Can you work these out from the model? Positions are in its coordinate system, mm. Face numbers are marked on the shaded views. A direction names the side the tool comes from. Coordinates: 2 decimals unless noted, no trailing zeros. Order: outer loops, then holes, each group sorted by start corner. A loop starts at its lowest first (then second) coordinate and runs counter-clockwise, first axis right, second up.
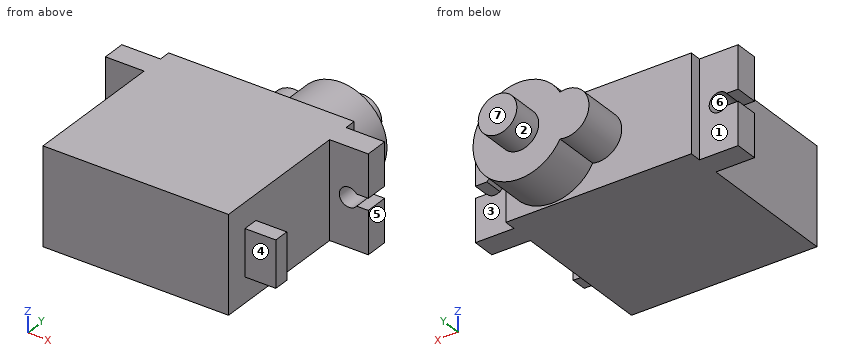
Autodesk Inventor part; units mm, degrees
ref_plane "YZ Plane" through (0, 0, 0) normal (1, 0, 0) x (0, 1, 0)
ref_plane "XZ Plane" through (0, 0, 0) normal (0, 1, 0) x (-1, 0, 0)
ref_plane "XY Plane" through (0, 0, 0) normal (0, 0, 1) x (1, 0, 0)
sketch "草圖1" plane through (0, 0, 0) normal (0, 0, 1) x (1, 0, 0)
  line L0 (-18, -14.5) -> (6, -14.5)
  line L1 (6, -14.5) -> (6, -33)
  line L2 (6, -33) -> (-18, -33)
  line L3 (-18, -33) -> (-18, -14.5)
  line L4 (-23, -11.5) -> (11, -11.5)
  line L5 (11, -11.5) -> (11, -14.5)
  line L6 (11, -14.5) -> (-23, -14.5)
  line L7 (-23, -14.5) -> (-23, -11.5)
  line L8 (6, -11.5) -> (-18, -11.5)
  line L9 (-18, -11.5) -> (-18, -10)
  line L10 (-18, -10) -> (6, -10)
  line L11 (6, -10) -> (6, -11.5)
  line L12 (6, -10) -> (-9, -10)
  line L13 (-9, -10) -> (-9, -4)
  line L14 (-9, -4) -> (6, -4)
  line L15 (6, -4) -> (6, -10)
  line L16 (2.5, -4) -> (-2.5, -4)
  line L17 (-2.5, -4) -> (-2.5, 0)
  line L18 (-2.5, 0) -> (2.5, 0)
  line L19 (2.5, 0) -> (2.5, -4)
  point P0 (0, 0)
  point P1 (-6, -14.5)
  point P2 (-6, -11.5)
  point P3 (0, -4)
  point P4 (-18, -11.5)
  point P5 (6, -14.5)
  point P6 (0, 0)
  dimension "d0" = 24
  dimension "d1" = 18.5
  dimension "d2" = 34
  dimension "d3" = 3
  dimension "d4" = 1.5
  dimension "d5" = 6
  dimension "d6" = 9
  dimension "d7" = 5
  dimension "d8" = 4
  dimension "d9" = 6
extrude "擠出1" add sketch "草圖1" along normal mid plane 12.5 contours L6 L7 L4 L5 L0 | L0 L1 L2 L3 | L9 L10 L11 L4
sketch "草圖2" plane through (-18, -10, 6.25) normal (0, 1, 0) x (1, 0, 0)
  circle A0 centre (18, 6.25) radius 6
  circle A1 centre (12, 6.25) radius 3
  line L0 (0, 12.5) -> (0, 0) construction
  point P0 (9, 6.25)
  point P1 (0, 6.25)
  point P2 (12.75, 9.1547)
  point P3 (12.75, 3.3453)
  dimension "d13" = 12
  dimension "d14" = 9
extrude "擠出2" add sketch "草圖2" along normal blind 6
sketch "草圖3" plane through (-18, -4, 6.25) normal (0, 1, 0) x (1, 0, 0)
  circle A0 centre (18, 6.25) radius 2.5
  dimension "d17" = 5
extrude "擠出3" add sketch "草圖3" along normal blind 4
sketch "草圖4" plane through (-23, -11.5, 6.25) normal (0, 1, 0) x (1, 0, 0)
  line L0 (0, 12.5) -> (0, 0) construction
  line L1 (5, 0) -> (0, 0) construction
  line L2 (5, 12.5) -> (5, 0) construction
  line L3 (0, 12.5) -> (5, 12.5) construction
  line L4 (0, 6.25) -> (5, 6.25) construction
  circle A0 centre (2.5, 6.25) radius 1.25
  line L5 (0, 12.5) -> (0, 0)
  line L6 (0, 7) -> (1.5, 7)
  line L7 (1.5, 7) -> (1.5, 5.5)
  line L8 (1.5, 5.5) -> (0, 5.5)
  line L9 (0, 5.5) -> (0, 7)
  line L10 (0, 9.2582) -> (34, 9.2582) construction
  line L11 (34, 12.5) -> (34, 0)
  line L12 (17, 9.2582) -> (17, 6.5712) construction
  circle A1 centre (31.5, 6.25) radius 1.25
  line L13 (34, 7) -> (32.5, 7)
  line L14 (32.5, 7) -> (32.5, 5.5)
  line L15 (32.5, 5.5) -> (34, 5.5)
  line L16 (34, 5.5) -> (34, 7)
  point P0 (23, 6.25)
  point P1 (0, 5.5)
  point P2 (1.5, 7)
  point P3 (34, 6.25)
  dimension "d20" = 2.5
  dimension "d21" = 1.5
  dimension "d22" = 14.5
extrude "擠出4" cut sketch "草圖4" against normal up to surface (3 mm away)
sketch "草圖5" plane through (6, -33, 6.25) normal (1, 0, 0) x (0, 0, -1)
  line L0 (12.5, 18.5) -> (0, 18.5) construction
  line L1 (0, 0) -> (0, 18.5) construction
  line L2 (12.5, 0) -> (0, 0) construction
  line L3 (12.5, 18.5) -> (12.5, 0) construction
  line L4 (0, 18.5) -> (0, 0) construction
  line L5 (0, 5) -> (3.25, 5) construction
  line L6 (3.25, 5) -> (9.25, 5)
  line L7 (9.25, 5) -> (9.25, 3)
  line L8 (9.25, 3) -> (3.25, 3)
  line L9 (3.25, 3) -> (3.25, 5)
  line L10 (3.25, 5) -> (9.25, 5)
  line L11 (9.25, 5) -> (12.5, 5) construction
  point P0 (6.25, 33)
  dimension "d25" = 6
  dimension "d26" = 13.5
  dimension "d27" = 3
extrude "擠出5" add sketch "草圖5" along normal blind 4
properties part number "MG90_II"
1. Imagine slicing it at C-C on x = 0. Please give me the cut outline in (y, z), then the cut area to 4 significant figures.
Completed:
outline: (-33, -6.25) - (-10, -6.25) - (-10, -6) - (-4, -6) - (-4, -2.5) - (0, -2.5) - (0, 2.5) - (-4, 2.5) - (-4, 6) - (-10, 6) - (-10, 6.25) - (-33, 6.25) - close
area: 379.5 mm2
2. I'm going to push flat-ended pins straight in: pin 1 (4 mm diameter, centred on x = -21.5, z = -1, fed in from +Y); pin 2 (0.6 mm diameter, centred on x = 7, y = -28.5, fed in from -Z); pin 3 (0.6 mm diameter, centred on y = -29, z = 0.5, fed in from +X). Where does each tip first touch, or does it pass through?
Completed:
pin 1: stops at y = -11.5
pin 2: stops at z = -3
pin 3: stops at x = 10
3. Thinking about a two-plate mould opening in X: for the marked faces 5, 6 and 7, which applies, pulls with the +X half, pulls with the -X half, needs draft (parallel to the pull), parting line crosses it, or undercut?
Completed:
face 5: pulls with the +X half
face 6: undercut
face 7: needs draft
4. Please list where these lines run through material, in increasing order: probe 1 along Z at (x, y) = (8.5, -13.05); probe 2 along Y at (x, z) = (-2, -5.25); probe 3 along Y at (x, z) = (-17.5, -5.25).
Completed:
probe 1: z = -6.25 to -1.25, 1.25 to 6.25
probe 2: y = -33 to -4
probe 3: y = -33 to -10
5. Imagine slicing it at B-B on x = -20.5. Please give me the cut outline in (y, z).
Completed:
outline: (-14.5, -6.25) - (-11.5, -6.25) - (-11.5, -1.25) - (-14.5, -1.25) - close; (-14.5, 1.25) - (-11.5, 1.25) - (-11.5, 6.25) - (-14.5, 6.25) - close
6. Imagine slicing it at A-A on x = 8.5. Please give me the cut outline in (y, z), then the cut area to 3 significant figures.
Completed:
outline: (-30, -3) - (-28, -3) - (-28, 3) - (-30, 3) - close; (-14.5, -6.25) - (-11.5, -6.25) - (-11.5, -1.25) - (-14.5, -1.25) - close; (-14.5, 1.25) - (-11.5, 1.25) - (-11.5, 6.25) - (-14.5, 6.25) - close
area: 42.0 mm2
7. On a 3-axis mill with a long thin cutter (end or side, diameter ignored), from which of +Z, -Z, +X, -X, +Y, -Y can I reach the whole of each face in a straight line? I mean the marked faces 1, 2, 3 and 4. Say none if no direction works.
Completed:
face 1: +Z, -Z, -X, +Y
face 2: +Y
face 3: +Z, -Z, +X, +Y
face 4: +Z, -Z, +X, -Y
8. Imagine slicing it at D-D on y = -22. Please give me the cut outline in (x, z).
Completed:
outline: (-18, -6.25) - (6, -6.25) - (6, 6.25) - (-18, 6.25) - close
